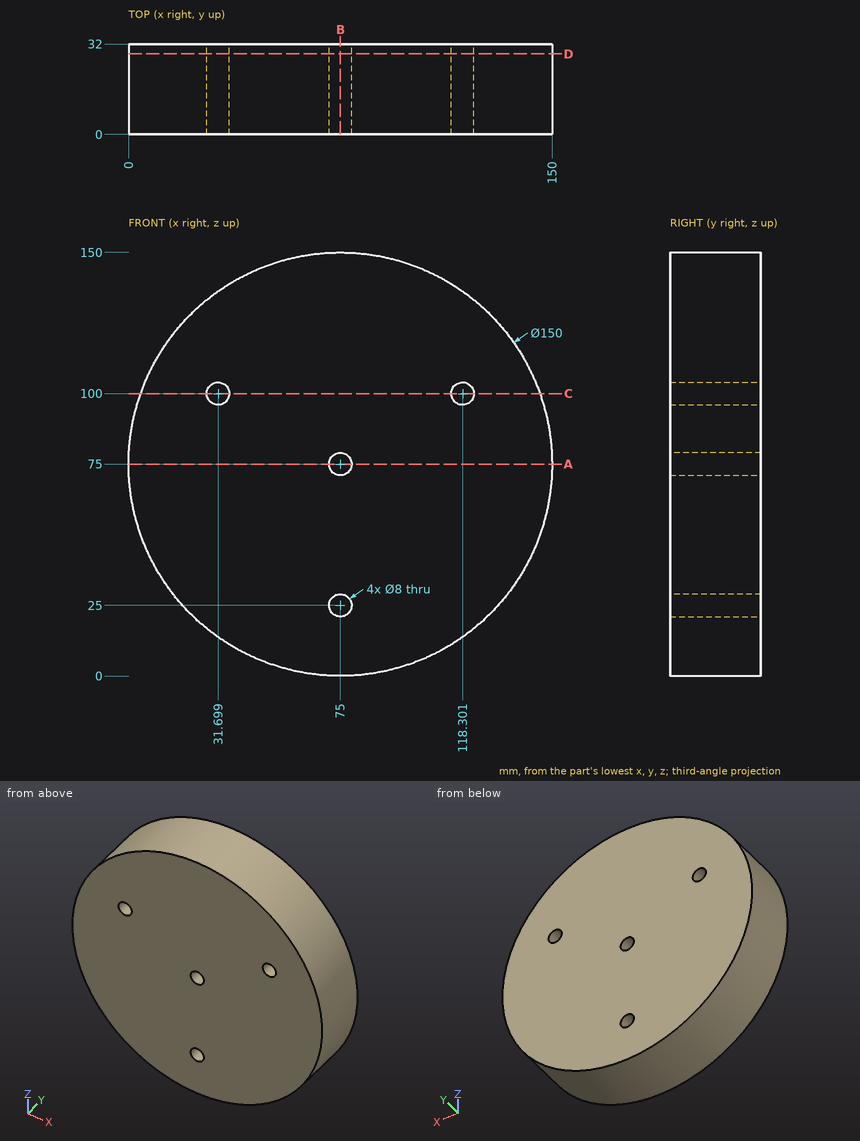
For this review, use the dimensioned drawing (mm, ordinates from the lowest corner) and the shaded views. Give positions to 0.01 mm unless a question says otherwise; leave off trailing zeros. Order: outer loops, then holes, each group sorted by start corner. A loop starts at its lowest first (then second) coordinate and runs counter-clockwise, first axis right, second up. Notation, with made-up numbers: (14, 71.25) - (72, 71.25) arc R34 ccw to (72, 106.25) - close; hole circle Ø5 at (-34.5, -19). An arc over 180 degrees is marked (long way). Use a Markdown table: item, result. Add a question column.
(1) Add section B-B on x = 75. Give the boundary of the cut face in (y, z).
(2) Clearance check with flat-ended pins moving along their axes: P1, Ø1.5, axis at x = 66.5, y = 13, coming from the -Z side; P2, Ø1.5, axis at y = 6.5, z = 34.5, coming from the -X side; P3, Ø6, axis at y = 16.5, z = 71.5, coming from the -X side. State where each tip first meets the part, or that it passes through.
(3) Add section C-C on z = 100. Give the boundary of the cut face in (x, y).
(4) Wall thickness on probe 1 along Z at (x, y) = (78.5, 18) (1 decimal); probe 2 along X at (y, z) = (9, 75); probe 3 along X at (y, z) = (17, 100): over which ranges is each line inside the solid? List them lowest first. Write a range as [from, to].
(5) Add section D-D on y = 28.5. Give the boundary of the cut face in (x, z), then the cut area to 3 significant figures.
(6) Add section A-A on z = 75. Give the boundary of the cut face in (x, y).
Report:
| question | item | result |
|---|---|---|
| 1 | outline | (0, 0) - (32, 0) - (32, 21) - (0, 21) - close; (0, 29) - (32, 29) - (32, 71) - (0, 71) - close; (0, 79) - (32, 79) - (32, 150) - (0, 150) - close |
| 2 | P1 | stops at z = 0.4 |
| 2 | P2 | stops at x = 11.4 |
| 2 | P3 | stops at x = 0 |
| 3 | outline | (4.29, 0) - (27.7, 0) - (27.7, 32) - (4.29, 32) - close; (35.7, 0) - (114.3, 0) - (114.3, 32) - (35.7, 32) - close; (122.3, 0) - (145.71, 0) - (145.71, 32) - (122.3, 32) - close |
| 4 | probe 1 | z = [0.1, 23.1], [26.9, 73.1], [76.9, 149.9] |
| 4 | probe 2 | x = [0, 71], [79, 150] |
| 4 | probe 3 | x = [4.29, 27.7], [35.7, 114.3], [122.3, 145.71] |
| 5 | outline | circle Ø150 at (75, 75); hole circle Ø8 at (31.7, 100); hole circle Ø8 at (75, 25); hole circle Ø8 at (75, 75); hole circle Ø8 at (118.3, 100) |
| 5 | area | 17,500 mm² |
| 6 | outline | (0, 0) - (71, 0) - (71, 32) - (0, 32) - close; (79, 0) - (150, 0) - (150, 32) - (79, 32) - close |
